Drawing for the job (mm, zero at the part's lowest x, y, z). A direction names the side the tool comes from. Round coordinates to 2 decimals unless told otherwise and drop trailing zeros. Loops run counter-clockwise (first coordinate to the right, second up) from the corner with the lowest first, then second, coordinate; pieces in that order, holes last. Notation, with made-up numbers: M 43.25,50 L 93.25,50 A17 ccw 93.25,54 Z; hole C -20,52 d11. An arc over 180 degrees is marked long. Answer in a Markdown table with one row per item.
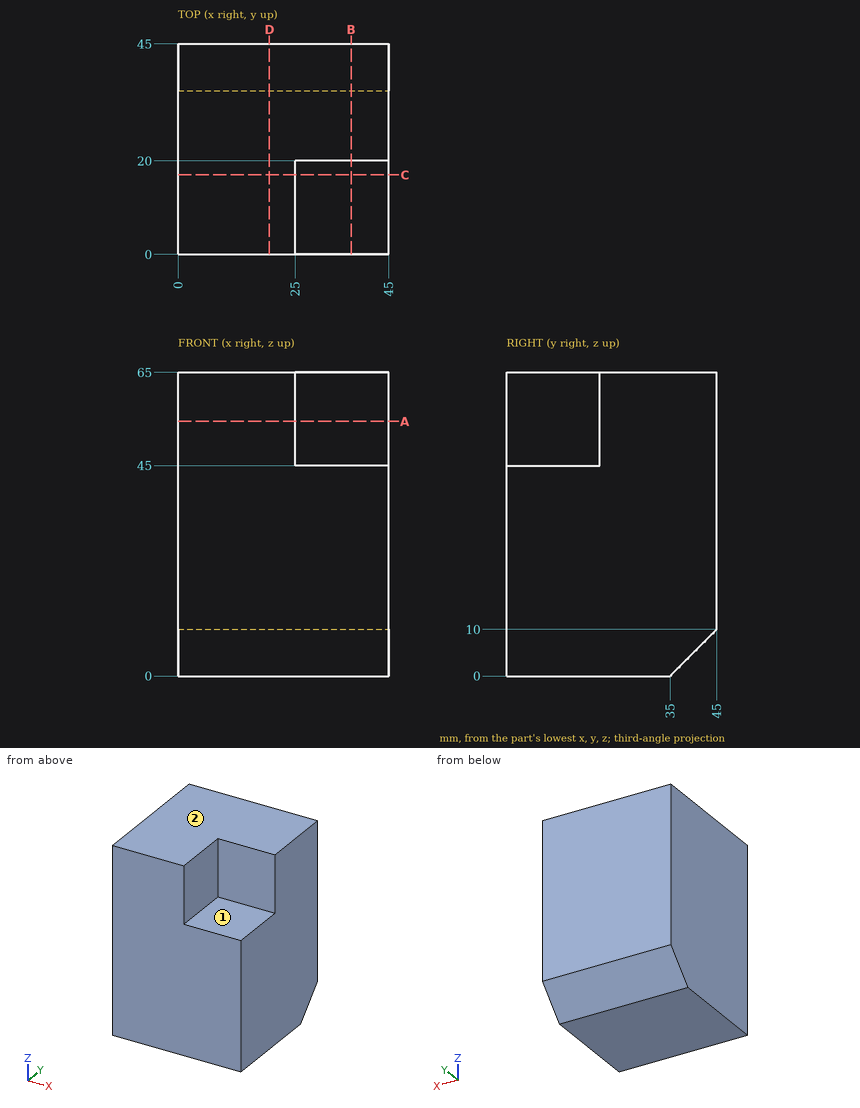
1. Saw through at B-B (x = 37). Write the cut outline in (y, z), and give its area (4 significant figures).
Verdict:
| item | result |
|---|---|
| outline | M 0,0 L 35,0 L 45,10 L 45,65 L 20,65 L 20,45 L 0,45 Z |
| area | 2,475 mm² |
2. Tool access for the marked faces 1 and 2: list every direction of +Z, -Z, +X, -X, +Y, -Y with a clear straight run to the whole face (end or side of a thin tool).
Verdict:
| item | result |
|---|---|
| face 1 | +Z, +X, -Y |
| face 2 | +Z, +X, -X, +Y, -Y |
3. Wall check: probe 1 along X at (y, z) = (3.5, 55); probe 2 along Z at (x, y) = (38, 16); probe 3 along Z at (x, y) = (36, 41). Give the ranges that are in metal, low to high.
Verdict:
| item | result |
|---|---|
| probe 1 | x = 0 to 25 |
| probe 2 | z = 0 to 45 |
| probe 3 | z = 6 to 65 |
4. Saw through at D-D (x = 19.5). Write the cut outline in (y, z).
Verdict:
| item | result |
|---|---|
| outline | M 0,0 L 35,0 L 45,10 L 45,65 L 0,65 Z |
5. Saw through at A-A (z = 54.5). Write the cut outline in (x, y).
Verdict:
| item | result |
|---|---|
| outline | M 0,0 L 25,0 L 25,20 L 45,20 L 45,45 L 0,45 Z |
6. Pin check, flat tips, straight feed: pin 1 (6 mm diameter, centred on x = 36.5, y = 12.5, fed in from +Z); pin 2 (10 mm diameter, centred on y = 7.5, z = 59.5, fed in from +X). Stop position of each tip, or through.
Verdict:
| item | result |
|---|---|
| pin 1 | stops at z = 45 |
| pin 2 | stops at x = 25 |
7. Saw through at C-C (y = 17). Write the cut outline in (x, z), and give its area (4 significant figures).
Verdict:
| item | result |
|---|---|
| outline | M 0,0 L 45,0 L 45,45 L 25,45 L 25,65 L 0,65 Z |
| area | 2,525 mm² |
